Check sheet for the modelled part. Datum: model origin and axes. Units: mm. A direction names the side the tool comes from. Round coordinates to 2 decimals unless told otherwise and drop trailing zeros. Write each loop counter-clockwise with the first axis right and the second up, starting at its lowest first coordinate (ties: lowest second). Pieces come first, ordered by that corner, then holes. Notation, with made-up numbers: (14, -28) -> (63, -28) arc R21 cw to (63, 4) -> close; hole circle Ø9 at (62.25, 7). An arc over 180 degrees is marked (long way). Put each result on its own line as item: value. Start each with the question number.
Autodesk Inventor part; units mm, degrees
ref_plane "Work Plane1" through (-19.4127, -19.4127, 20.695) normal (0, 0, -1) x (0, 1, 0)
ref_plane "YZ Plane" through (0, 0, 0) normal (1, 0, 0) x (0, 1, 0)
ref_plane "XZ Plane" through (0, 0, 0) normal (0, 1, 0) x (-1, 0, 0)
sketch "Sketch1" plane through (0, 0, 0) normal (0, 0, 1) x (1, 0, 0)
  circle A0 centre (0, 0) radius 31.75
  line L0 (25.4, 38.1) -> (25.4, -38.1)
  circle A1 centre (20.7166, 31.75) radius 2.3813
  line L1 (14.986, 531.4221) -> (14.986, -382.9779)
  line L2 (-25.4, 38.1) -> (25.4, 38.1)
  circle A2 centre (-20.7166, 31.75) radius 2.3813
  line L3 (-25.4, -38.1) -> (-25.4, 38.1)
  circle A3 centre (-20.7166, -31.75) radius 2.3813
  line L4 (25.4, -38.1) -> (-25.4, -38.1)
  circle A4 centre (20.7166, -31.75) radius 2.3813
  circle A5 centre (0, 0) radius 31.75
  point P0 (0, 0)
  point P1 (25.4, -19.05)
  point P2 (-25.4, -19.05)
  point P3 (-25.4, 19.05)
  point P4 (25.4, 19.05)
ref_plane "Work Plane1" through (-19.4127, -19.4127, 20.695) normal (0, 0, -1) x (0, 1, 0)
extrude "Extrusion1" add sketch "Sketch1" along normal up to surface (20.695 mm away) contours A0 L1 L2 L0 | L0 L4 L1 A0 | A0 L3 L2 L1 | L1 L4 L3 A0
sketch "Sketch2" plane through (0, 0, 20.695) normal (0, 0, 1) x (1, 0, 0)
  arc A0 (-25.4, -19.05) -> (25.4, -19.05) centre (0, 0) ccw
  line L0 (25.4, 38.1) -> (25.4, -38.1)
  arc A1 (25.4, 19.05) -> (-25.4, 19.05) centre (0, 0) ccw
  line L1 (-25.4, -38.1) -> (-25.4, 38.1)
  circle A2 centre (-15.5, -15.5) radius 1.6449
  circle A3 centre (15.5, 15.5) radius 1.6449
  circle A4 centre (0, 0) radius 7.9375
  point P0 (0, 0)
  dimension "d2" = 15.875
extrude "Extrusion2" add sketch "Sketch2" against normal blind 6.35
fillet "Fillet1" radius 3.175 8 edges at (-25.4, -19.05, 7.1725) (-25.4, 19.05, 7.1725) (-25.4, 38.1, 10.3475) (25.4, 38.1, 10.3475) (25.4, -38.1, 10.3475) (-25.4, -38.1, 10.3475) (25.4, 19.05, 7.1725) (25.4, -19.05, 7.1725)
properties part number "Printed Encoder Mount"
1. Material ranges on L1, parallel to Y at x = -1, z = 12.75; L2, parallel to Y at x = -22, z = 16; L3, parallel to Y at x = -15.5, z = 17, recorded low to high. Write a range as [from, to].
2. Section check B-B, the plane y = 0. Enter the section's corners in (x, z) (1 decimal).
3. Section check D-D, the plane y = 15.5. Enter the section's corners in (x, z) (3 decimals), then the cut area to 3 significant figures.
4. Section check A-A, the plane z = 8.5. Enter the section's corners in (x, y) (3 decimals).
5. Gauge pin test, flat ends, axial feed: P1, Ø15, axis at x = -11, y = -9, coming from the -Z side (3 decimals); P2, Ø8, axis at y = 6, z = 7.5, coming from the +X side; P3, Ø7.5, axis at x = 20.72, y = -31.75, coming from the +Z side (3 decimals). Record the tip position at first contact, or that the pin passes through.
6. Draft check along X on faces 3 (the flat face through (0, 33, 0)), 4 (the flat face through (-25.4, 0, 15)), 5 (the cylindrical face through (-13.93, -15.01, 17.56)). Enter one of: released by +X, released by -X, zero draft, split by the parting line, or undercut.
7. Access from +Z, -Z, +X, -X, +Y, -Y to the whole of each face (thin tool, end or side, straight path). Record for faces 1 (the cylindrical face through (-23.533, -24.048, 7.273)), 2 (the cylindrical face through (17.07, 15.99, 17.56)).
Reply:
1. L1: y = [-38.1, -31.73], [31.73, 38.1]
1. L2: y = [-38.1, -33.76], [-29.74, 29.74], [33.76, 38.1]
1. L3: y = [-38.1, -17.14], [-13.86, 38.1]
2. outline: (-25.4, 14.3) -> (-7.9, 14.3) -> (-7.9, 20.7) -> (-25.4, 20.7) -> close; (7.9, 14.3) -> (25.4, 14.3) -> (25.4, 20.7) -> (7.9, 20.7) -> close
3. outline: (-25.4, 14.345) -> (13.855, 14.345) -> (13.855, 20.695) -> (-25.4, 20.695) -> close; (17.145, 14.345) -> (25.4, 14.345) -> (25.4, 20.695) -> (17.145, 20.695) -> close
3. area: 302 mm2
4. outline: (-25.4, -34.925) arc R3.175 ccw to (-22.225, -38.1) -> (22.225, -38.1) arc R3.175 ccw to (25.4, -34.925) -> (25.4, -26.941) arc R3.175 ccw to (20.205, -24.492) arc R31.75 cw to (-20.205, -24.492) arc R3.175 ccw to (-25.4, -26.941) -> close; (-25.4, 26.941) arc R3.175 ccw to (-20.205, 24.492) arc R31.75 cw to (20.205, 24.492) arc R3.175 ccw to (25.4, 26.941) -> (25.4, 34.925) arc R3.175 ccw to (22.225, 38.1) -> (-22.225, 38.1) arc R3.175 ccw to (-25.4, 34.925) -> close; hole circle Ø4.763 at (-20.717, -31.75); hole circle Ø4.763 at (-20.717, 31.75); hole circle Ø4.763 at (20.717, -31.75); hole circle Ø4.763 at (20.717, 31.75)
5. P1: stops at z = 14.345
5. P2: passes through
5. P3: stops at z = 20.695
6. face 3: zero draft
6. face 4: released by -X
6. face 5: undercut
7. face 1: -Z
7. face 2: +Z, -Z
